The model under review builds one solid part; all positions refer to its coordinate system, in mm. A direction names the side the tool comes from. Round coordinates to 2 decimals unless told otherwise and drop trailing zeros. Write each loop counter-clockwise with the first axis right and the second up, starting at its lowest first coordinate (ties: lowest second). Pieces come first, ordered by that corner, then holes. Notation, with made-up numbers: (-34.5, 61.25) - (-0.5, 61.25) arc R20 cw to (-0.5, 80.25) - close; hole circle Ø8 at (38.5, 35.25). An arc over 180 degrees is marked (long way). One line per question, with ' | ' between items. Start each with the question number.
```python
from build123d import *

# Parameters (mm, degrees)
BOSS_EXTRUDE1_DEPTH = 19.05
SKETCH2_W           = 12.7
SKETCH2_H           = 49.430607356
CUT_EXTRUDE1_DEPTH  = 81.742636051
SKETCH3_R           = 3.1877
CUT_EXTRUDE2_DEPTH  = 91.02678768
CUT_EXTRUDE3_DEPTH  = 12.7
SKETCH4_3_R         = 3.1877
CUT_EXTRUDE5_DEPTH  = 107.4453968


with BuildPart() as part:
    # Sketch1 → Boss-Extrude1 (new body)
    with BuildSketch(Plane.XY):
        Polygon((0, 0), (0, 25.4), (86.935303163, 25.4), (101.6, 0), align=None)
    extrude(amount=BOSS_EXTRUDE1_DEPTH)

    # Sketch2 → Cut-Extrude1 (cut, through all)
    with BuildSketch(Plane(origin=(67.951108029, 39.231590512, 0), x_dir=(0, 0, -1), z_dir=(0.8660254037844359, 0.5000000000000048, 0))):
        with Locations((-9.525, -49.360910003)):
            Rectangle(SKETCH2_W, SKETCH2_H)
    extrude(amount=-CUT_EXTRUDE1_DEPTH, mode=Mode.SUBTRACT)

    # Sketch3 → Cut-Extrude2 (cut, through all)
    with BuildSketch(Plane(origin=(76.2, 43.994090512, 0), x_dir=(0, 0, -1), z_dir=(0.8660254037844359, 0.5000000000000048, 0))):
        with Locations(Location((-9.525, -36.135303163, 0), (0, 0, 90))):
            Circle(SKETCH3_R)
    extrude(amount=-CUT_EXTRUDE2_DEPTH, mode=Mode.SUBTRACT)

    # Sketch4 → Cut-Extrude3 (cut)
    with BuildSketch(Plane(origin=(0, 25.4, 0), x_dir=(1, 0, 0), z_dir=(0, 1, 0))):
        with BuildLine():
            Line((12.7, -3.175), (44.45, -3.175))
            ThreePointArc((44.45, -3.175), (50.8, -9.525), (44.45, -15.875))
            Line((44.45, -15.875), (12.7, -15.875))
            ThreePointArc((12.7, -15.875), (6.35, -9.525), (12.7, -3.175))
        make_face()
    extrude(amount=-CUT_EXTRUDE3_DEPTH, mode=Mode.SUBTRACT)

    # Sketch4_3 → Cut-Extrude5 (cut, through all)
    with BuildSketch(Plane(origin=(0, 25.4, 0), x_dir=(1, 0, 0), z_dir=(0, 1, 0))):
        with Locations(Location((12.7, -9.525, 0), (0, 0, 270))):
            Circle(SKETCH4_3_R)
        with Locations(Location((44.45, -9.525, 0), (0, 0, 270))):
            Circle(SKETCH4_3_R)
    extrude(amount=-CUT_EXTRUDE5_DEPTH, mode=Mode.SUBTRACT)


solid = part.part
```
1. Wall thickness on line 1 along Z through (x, y) = (24, 17.75) (3 decimals); line 2 along X through (y, z) = (14.5, 14.5); line 3 along Y through (x, z) = (40.5, 13.25): over which ranges is each line inside the solid? List them lowest first. Write a range as [from, to].
2. Clearance check with flat-ended pins moving along their axes: P1, Ø1.5, axis at y = 6.5, z = 12, coming from the +X side; P2, Ø1, axis at x = 81, z = 7.5, coming from the -Y side; P3, Ø4, axis at y = 20.5, z = 5, coming from the +X side. State where each tip first meets the part, or that it passes through.
3. Add section A-A, the plane y = 4.25. Write out the cut boundary in (x, z) (3 decimals).
4. The part is to be moulded in two halves that separate along X. For faces 1 (the face through (53, 25.4, 9)), 2 (the face through (65, 9.07, 9.61)), 3 (the face through (0, 13, 9)), 4 (the face through (92.536, 15.7, 9.392)), say which applies: pulls with the +X half, pulls with the -X half, needs draft (parallel to the pull), parting line crosses it, or undercut.
5. Add section B-B, the plane x = 83. Write out the cut boundary in (y, z) (3 decimals).
6. Add section C-C, the plane z = 14.75. Write out the cut boundary in (x, y).
7. Add section D-D, the plane x = 64.5. Write out the cut boundary in (y, z) (3 decimals).
8. Machinability: for faces 5 (the face through (52, 13, 19.05)), 6 (the face through (29, 19, 15.875)), 7 (the face through (84.218, 11.057, 9.614)), which of the approach directions +Z, -Z, +X, -X, +Y, -Y give a long, thin tool a straight path to every point of the face, cutting with its end or side? Answer none if there is none.
Geometry check:
1) line 1: z = [0, 3.175], [15.875, 19.05] | line 2: x = [0, 8.75], [48.4, 74.41], [82.23, 93.23] | line 3: y = [0, 12.7]
2) P1: stops at x = 98.28 | P2: stops at y = 15.76 | P3: stops at x = 90.92
3) outline: (0, 0) - (99.146, 0) - (99.146, 19.05) - (0, 19.05) - close; hole circle Ø6.375 at (12.7, 9.525); hole circle Ø6.375 at (44.45, 9.525); hole (56.652, 3.175) - (88.148, 3.175) - (88.148, 15.875) - (56.652, 15.875) - close
4) face 1: needs draft | face 2: undercut | face 3: pulls with the -X half | face 4: pulls with the +X half
5) outline: (0, 0) - (25.4, 0) - (25.4, 19.05) - (0, 19.05) - (0, 15.875) - (13.166, 15.875) - (13.166, 3.175) - (0, 3.175) - close
6) outline: (0, 0) - (49.29, 0) - (80.27, 17.89) - (90.6, 0) - (101.6, 0) - (86.94, 25.4) - (48.06, 25.4) - (48.06, 12.7) - (9.09, 12.7) - (9.09, 25.4) - (0, 25.4) - close
7) outline: (0, 0) - (25.4, 0) - (25.4, 19.05) - (0, 19.05) - (0, 15.875) - (8.781, 15.875) - (8.781, 3.175) - (0, 3.175) - close
8) face 5: +Z, +X, -X, +Y, -Y | face 6: +Y | face 7: -Y
